```python
from build123d import *

# Parameters (mm, degrees)
SKETCH1_W           = 37
SKETCH1_H           = 37
BOSS_EXTRUDE1_DEPTH = 1637.5
SKETCH2_W           = 10
SKETCH2_H           = 20
CUT_EXTRUDE1_DEPTH  = 40
SKETCH3_W           = 21
SKETCH3_H           = 2
CUT_EXTRUDE2_DEPTH  = 20
SKETCH4_W           = 10
SKETCH4_H           = 41
CUT_EXTRUDE3_DEPTH  = 1639.476807892
CUT_EXTRUDE4_DEPTH  = 20
SKETCH7_W           = 20
SKETCH7_H           = 20
CUT_EXTRUDE6_DEPTH  = 20
SKETCH8_W           = 4
SKETCH8_H           = 120
CUT_EXTRUDE7_DEPTH  = 22
SKETCH9_R           = 3
CUT_EXTRUDE8_DEPTH  = 22
LPATTERN1_COUNT     = 2
LPATTERN1_PITCH     = 190
LPATTERN2_COUNT     = 2
LPATTERN2_PITCH     = 800
SKETCH10_R          = 10
CUT_EXTRUDE9_DEPTH  = 1639.476807892
SKETCH11_R          = 10
CUT_EXTRUDE10_DEPTH = 1639.476807892


with BuildPart() as part:
    # Sketch1 → Boss-Extrude1 (new body)
    with BuildSketch(Plane(origin=(0, 0, 0), x_dir=(1, 0, 0), z_dir=(0, 1, 0))):
        with BuildLine():
            Line((0.5, 0), (39.5, 0))
            ThreePointArc((39.5, 0), (39.853553391, 0.146446609), (40, 0.5))
            Line((40, 0.5), (40, 39.5))
            ThreePointArc((40, 39.5), (39.853553391, 39.853553391), (39.5, 40))
            Line((39.5, 40), (0.5, 40))
            ThreePointArc((0.5, 40), (0.146446609, 39.853553391), (0, 39.5))
            Line((0, 39.5), (0, 0.5))
            ThreePointArc((0, 0.5), (0.146446609, 0.146446609), (0.5, 0))
        make_face()
        with Locations((20, 20)):
            Rectangle(SKETCH1_W, SKETCH1_H, mode=Mode.SUBTRACT)
    extrude(amount=BOSS_EXTRUDE1_DEPTH)

    # Sketch2 → Cut-Extrude1 (cut)
    with BuildSketch(Plane(origin=(40, 0, 0), x_dir=(0, 0, -1), z_dir=(1, 0, 0))):
        with Locations((35, 1627.5)):
            Rectangle(SKETCH2_W, SKETCH2_H)
        with Locations((5, 1627.5)):
            Rectangle(SKETCH2_W, SKETCH2_H)
    extrude(amount=-CUT_EXTRUDE1_DEPTH, mode=Mode.SUBTRACT)

    # Sketch3 → Cut-Extrude2 (cut)
    with BuildSketch(Plane(origin=(40, 0, 0), x_dir=(0, 0, -1), z_dir=(1, 0, 0))):
        with Locations((29.5, 1534)):
            Rectangle(SKETCH3_W, SKETCH3_H)
        with Locations((29.5, 1496)):
            Rectangle(SKETCH3_W, SKETCH3_H)
    extrude(amount=-CUT_EXTRUDE2_DEPTH, mode=Mode.SUBTRACT)

    # Sketch4 → Cut-Extrude3 (cut, through all)
    with BuildSketch(Plane.XY):
        with Locations((35, 20.5)):
            Rectangle(SKETCH4_W, SKETCH4_H)
        with Locations((5, 20.5)):
            Rectangle(SKETCH4_W, SKETCH4_H)
    extrude(amount=-CUT_EXTRUDE3_DEPTH, mode=Mode.SUBTRACT)

    # Sketch5 → Cut-Extrude4 (cut)
    with BuildSketch(Plane(origin=(40, 0, -40), x_dir=(1, 0, 0), z_dir=(0, 0, 1))):
        Polygon((-40, 190.5), (-20, 190.5), (-20, 231), (-30, 231), (-30, 211), (-40, 211), align=None)
        Polygon((-40, 380.5), (-20, 380.5), (-20, 421), (-30, 421), (-30, 401), (-40, 401), align=None)
        Polygon((-40, 570.5), (-20, 570.5), (-20, 611), (-30, 611), (-30, 591), (-40, 591), align=None)
        Polygon((-40, 760.5), (-20, 760.5), (-20, 801), (-30, 801), (-30, 781), (-40, 781), align=None)
    extrude(amount=CUT_EXTRUDE4_DEPTH, mode=Mode.SUBTRACT)

    # Sketch7 → Cut-Extrude6 (cut)
    with BuildSketch(Plane(origin=(40, 0, 0), x_dir=(0, 0, -1), z_dir=(1, 0, 0))):
        with Locations((30, 1033)):
            Rectangle(SKETCH7_W, SKETCH7_H)
    extrude(amount=-CUT_EXTRUDE6_DEPTH, mode=Mode.SUBTRACT)

    # Sketch8 → Cut-Extrude7 (cut)
    with BuildSketch(Plane(origin=(40, 0, 0), x_dir=(0, 0, -1), z_dir=(1, 0, 0))):
        with Locations((38, 119)):
            Rectangle(SKETCH8_W, SKETCH8_H)
    cut_extrude7 = extrude(amount=-CUT_EXTRUDE7_DEPTH, mode=Mode.SUBTRACT)

    # Sketch9 → Cut-Extrude8 (cut)
    with BuildSketch(Plane(origin=(0, 0, -1.5), x_dir=(-1, 0, 0), z_dir=(0, 0, -1))):
        with Locations((-28, 162.5)):
            Circle(SKETCH9_R)
        with Locations((-28, 78.5)):
            Circle(SKETCH9_R)
    cut_extrude8 = extrude(amount=-CUT_EXTRUDE8_DEPTH, mode=Mode.SUBTRACT)

    # LPattern1: Cut-Extrude7, Cut-Extrude8 ×2
    with Locations(*[(0, i * LPATTERN1_PITCH, 0) for i in range(1, LPATTERN1_COUNT)]):
        add(cut_extrude7, mode=Mode.SUBTRACT)
        add(cut_extrude8, mode=Mode.SUBTRACT)

    # LPattern2: Cut-Extrude7, Cut-Extrude8 ×2
    with Locations(*[(0, i * LPATTERN2_PITCH, 0) for i in range(1, LPATTERN2_COUNT)]):
        add(cut_extrude7, mode=Mode.SUBTRACT)
        add(cut_extrude8, mode=Mode.SUBTRACT)

    # Sketch10 → Cut-Extrude9 (cut, through all)
    with BuildSketch(Plane.XY):
        with Locations((20, 1577.5)):
            Circle(SKETCH10_R)
        with Locations((20, 1227.5)):
            Circle(SKETCH10_R)
    extrude(amount=-CUT_EXTRUDE9_DEPTH, mode=Mode.SUBTRACT)

    # Sketch11 → Cut-Extrude10 (cut, through all)
    with BuildSketch(Plane.ZY):
        with Locations((-25, 1467.5)):
            Circle(SKETCH11_R)
        with Locations((-25, 1217.5)):
            Circle(SKETCH11_R)
        with Locations((-25, 967.5)):
            Circle(SKETCH11_R)
    extrude(amount=-CUT_EXTRUDE10_DEPTH, mode=Mode.SUBTRACT)


solid = part.part
```
Geometry: final body of the model. Coordinates: model frame, mm. A direction names the side the tool comes from. Coordinates: 2 decimals unless noted, no trailing zeros. Answer as CSV lines item,"result". Start each with the question number.
Q1. Pin query (flat end, axial travel): P1, Ø1.6, axis at x = 1, y = 390, coming from the -Z side; P2, Ø0.8, axis at y = 12, z = -39.5, coming from the -X side; P3, Ø10, axis at x = 29.5, z = -26, coming from the -Y side; P4, Ø12, axis at x = 32.5, z = -35, coming from the +Y side. Return the tip coordinate at first contact, or that it passes through.
Q2. Mould query, pull axis Z, two halves, no side actions, for faces 1 (the flat face through (1.5, 828, -20)), 2 (the flat face through (20, 797, -1.5)), 3 (the flat face through (0, 828, -20)), 4 (the flat face through (20, 797, 0)). Classes: released by +Z, released by -Z, zero draft, split by the parting line, or undercut.
Q3. Line query: line 1 (Z direction, x = 39, y = 1467); line 2 (X direction, y = 1577.5, z = -0.85); line 3 (X direction, y = 237, z = -4). Output: solid intervals per line, ascending. Write a range as from..to.
Q4. Reachability of faces 5 (the flat face through (20.3, 797.4, -40)), 6 (the flat face through (24, 797, -38.5)) from +Z, -Z, +X, -X, +Y, -Y: full face, straight path, thin tool, end or side. Return the list, or none.
Findings below:
1,P1,"stops at z = -20"
1,P2,"stops at x = 10"
1,P3,"passes through"
1,P4,"stops at y = 1617.5"
2,face 1,"undercut"
2,face 2,"undercut"
2,face 3,"zero draft"
2,face 4,"released by +Z"
3,line 1,"z = -40..-34.99, -15.01..0"
3,line 2,"x = 0..10, 30..40"
3,line 3,"x = 0..1.5, 38.5..40"
4,face 5,"-Z, +X, -X, +Y, -Y"
4,face 6,"+Y, -Y"
